Geometry: final body of the model. Coordinates: model frame, mm. Face numbers are marked on the shaded views. Give positions to 0.01 mm unless a question says otherwise; leave off trailing zeros. Order: outer loops, then holes, each group sorted by start corner. A loop starts at its lowest first (then second) coordinate and runs counter-clockwise, first axis right, second up. Notation, with made-up numbers: (66.5, -25) - (75.5, -25) arc R16 ccw to (75.5, -7) - close; hole circle Ø11 at (-10, 86). An arc over 180 degrees is marked (long way). One line per item, written item: value.
```python
from build123d import *

# Parameters (mm, degrees)
CROQUIS1_R              = 18.4
SALIENTE_EXTRUIR1_DEPTH = 24.3
CROQUIS2_R              = 3
CROQUIS2_R_2            = 1.25
CORTAR_EXTRUIR1_DEPTH   = 5
CROQUIS3_R              = 1.25
CORTAR_EXTRUIR2_DEPTH   = 5
CORTAR_EXTRUIR3_START   = -5
CROQUIS6_R              = 18.4
CORTAR_EXTRUIR3_DEPTH   = 5
CROQUIS7_R              = 6
CORTAR_EXTRUIR4_DEPTH   = 1


with BuildPart() as part:
    # Croquis1 → Saliente-Extruir1 (new body)
    with BuildSketch(Plane.XY):
        Circle(CROQUIS1_R)
    extrude(amount=SALIENTE_EXTRUIR1_DEPTH)

    # Croquis2 → Cortar-Extruir1 (cut)
    with BuildSketch(Plane.XY.offset(24.3)):
        Circle(CROQUIS2_R)
        with Locations((0, 9.5)):
            Circle(CROQUIS2_R_2)
        with Locations((9.5, 0)):
            Circle(CROQUIS2_R_2)
        with Locations((0, -9.5)):
            Circle(CROQUIS2_R_2)
        with Locations((-9.5, 0)):
            Circle(CROQUIS2_R_2)
    extrude(amount=-CORTAR_EXTRUIR1_DEPTH, mode=Mode.SUBTRACT)

    # Croquis3 → Cortar-Extruir2 (cut)
    with BuildSketch(Plane(origin=(0, 0, 0), x_dir=(-1, 0, 0), z_dir=(0, 0, -1))):
        with Locations((-10, 0)):
            Circle(CROQUIS3_R)
        with Locations((0, 10)):
            Circle(CROQUIS3_R)
        with Locations((10, 0)):
            Circle(CROQUIS3_R)
        with Locations((0, -10)):
            Circle(CROQUIS3_R)
    extrude(amount=-CORTAR_EXTRUIR2_DEPTH, mode=Mode.SUBTRACT)

    # Croquis6 → Cortar-Extruir3 (cut)
    with BuildSketch(Plane.XY.offset(24.3).offset(CORTAR_EXTRUIR3_START)):
        Circle(CROQUIS6_R)
    extrude(amount=CORTAR_EXTRUIR3_DEPTH, mode=Mode.SUBTRACT)

    # Croquis7 → Cortar-Extruir4 (cut)
    with BuildSketch(Plane.XY.offset(19.3)):
        Circle(CROQUIS7_R)
    extrude(amount=-CORTAR_EXTRUIR4_DEPTH, mode=Mode.SUBTRACT)


solid = part.part
```
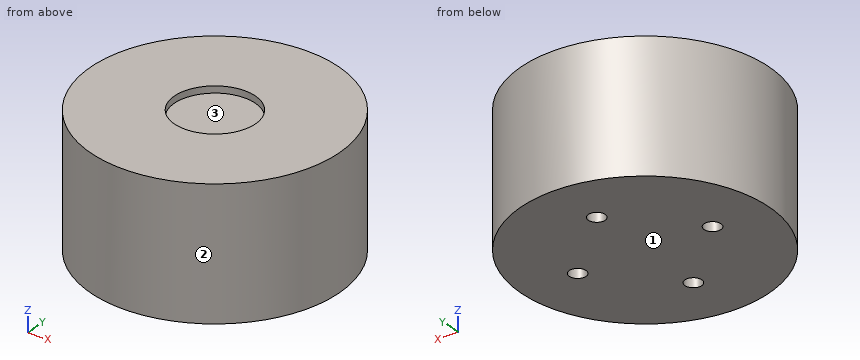
1) Material intervals for line 1 along Y through (x, z) = (0, 3); line 2 along Y through (x, z) = (0, 18.95); line 3 along Z through (x, y) = (1, 5), sorted ascending.
Answers below:
line 1: -18.4 to -11.25, -8.75 to 8.75, 11.25 to 18.4
line 2: -18.4 to -6, 6 to 18.4
line 3: 0 to 18.3
2) Section B-B, the plane y = -10. Return loops of the section in (x, z).
Answers below:
outline: (-15.45, 0) - (-1.25, 0) - (-1.25, 5) - (1.25, 5) - (1.25, 0) - (15.45, 0) - (15.45, 19.3) - (-15.45, 19.3) - close
3) Mould query, pull axis Y, two halves, no side actions, for the marked faces 1, 2 and 3. Classes: released by +Y, released by -Y, zero draft, split by the parting line, or undercut.
Answers below:
face 1: zero draft
face 2: split by the parting line
face 3: undercut
4) First-contact query: pin 1 (1.5 mm diameter, centred on x = 2, z = 2.5, fed in from -Y); pin 2 (2 mm diameter, centred on x = 10, y = 0, fed in from -Z); pin 3 (1 mm diameter, centred on y = 7, z = 8.5, fed in from +X). Flat tips, straight axial feed; report the tip coordinate or a pass-through.
Answers below:
pin 1: y = -18.36
pin 2: z = 5
pin 3: x = 17.21
5) Section C-C, the plane z = 12. Return loops of the section in (x, y), then the cut area to 3 significant figures.
Answers below:
outline: circle Ø36.8 at (0, 0)
area: 1,060 mm^2
6) Section A-A, the plane x = 0. Return loops of the section in (y, z).
Answers below:
outline: (-18.4, 0) - (-11.25, 0) - (-11.25, 5) - (-8.75, 5) - (-8.75, 0) - (8.75, 0) - (8.75, 5) - (11.25, 5) - (11.25, 0) - (18.4, 0) - (18.4, 19.3) - (6, 19.3) - (6, 18.3) - (-6, 18.3) - (-6, 19.3) - (-18.4, 19.3) - close
7) Section D-D, the plane x = -10.5. Return loops of the section in (y, z).
Answers below:
outline: (-15.11, 0) - (-1.15, 0) - (-1.15, 5) - (1.15, 5) - (1.15, 0) - (15.11, 0) - (15.11, 19.3) - (-15.11, 19.3) - close
